Could you check a few things on this drawing? It's one solid part, dimensions in mm from its lowest x, y, z. A direction names the side the tool comes from. Give positions to 0.01 mm unless a question says otherwise; leave off trailing zeros. Write each loop counter-clockwise with the first axis right and the second up, starting at its lowest first coordinate (ties: lowest second). Pieces come first, ordered by that corner, then holes. Notation, with made-up numbers: (-10.75, -19.75) - (12.25, -19.75) arc R15 cw to (12.25, 8.25) - close; hole circle Ø4 at (89.25, -32). An arc over 180 degrees is marked (long way). One line per item, written item: value. Start each with the question number.
1) I'm going to push flat-ended pins straight in: P1, Ø1.5, axis at y = 27, z = 61, coming from the +X side; P2, Ø6, axis at x = 68, z = 66, coming from the -Y side. Where does each tip first touch, or does it pass through?
2) Imagine slicing it at C-C on z = 69.5. Write out the boundary of the cut face in (x, y), plus the area to 3 significant figures.
3) On a 3-axis mill with a long thin cutter (end or side, diameter ignored), from which of +Z, -Z, +X, -X, +Y, -Y can I reach the whole of each face in a straight line? I mean the marked faces 1 and 2. Say none if no direction works.
4) Please list where these lines run through material, in increasing order: L1, parallel to Z at x = 13.5, y = 19.05; L2, parallel to X at y = 10.5, z = 51; L3, parallel to Y at x = 69.5, z = 46. Write a range as [from, to].
5) Imagine slicing it at B-B on z = 57.15. Write out the boundary of the cut face in (x, y), plus the area to 3 significant figures.
6) Imagine slicing it at A-A on y = 19.05. Write out the boundary of the cut face in (x, z).
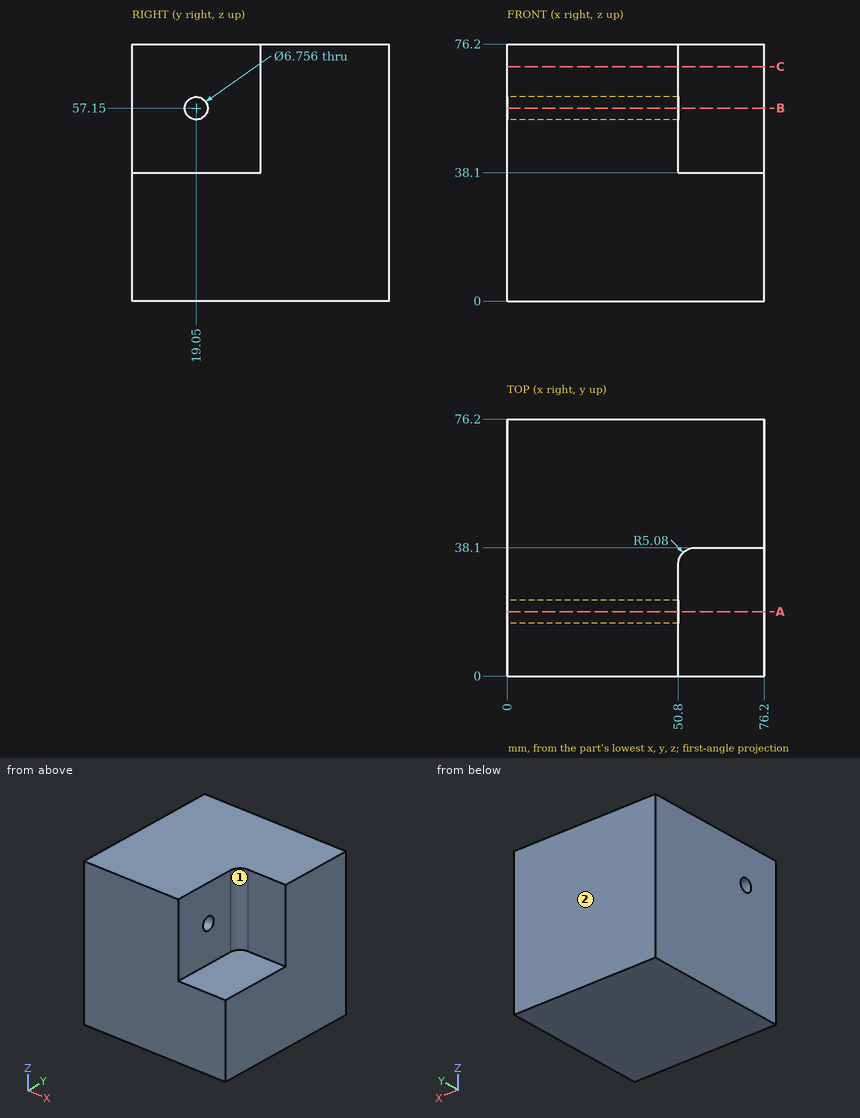
Numbers:
1. P1: x = 50.8
1. P2: y = 38.1
2. outline: (0, 0) - (50.8, 0) - (50.8, 33.02) arc R5.08 cw to (55.88, 38.1) - (76.2, 38.1) - (76.2, 76.2) - (0, 76.2) - close
2. area: 4,840 mm^2
3. face 1: +Z, +X, -Y
3. face 2: +Z, -Z, +X, -X, +Y
4. L1: [0, 53.77], [60.53, 76.2]
4. L2: [0, 50.8]
4. L3: [38.1, 76.2]
5. outline: (0, 0) - (50.8, 0) - (50.8, 15.67) - (0, 15.67) - close; (0, 22.43) - (50.8, 22.43) - (50.8, 33.02) arc R5.08 cw to (55.88, 38.1) - (76.2, 38.1) - (76.2, 76.2) - (0, 76.2) - close
5. area: 4,500 mm^2
6. outline: (0, 0) - (76.2, 0) - (76.2, 38.1) - (50.8, 38.1) - (50.8, 53.77) - (0, 53.77) - close; (0, 60.53) - (50.8, 60.53) - (50.8, 76.2) - (0, 76.2) - close
